Model file for the job. Use its own axes, mm. Face numbers are marked on the shaded views. A direction names the side the tool comes from. Round coordinates to 2 decimals unless told otherwise and drop trailing zeros. Loops run counter-clockwise (first coordinate to the right, second up) from the corner with the lowest first, then second, coordinate; pieces in that order, holes last. Notation, with made-up numbers: (-27, 43) - (31, 43) arc R16 cw to (31, 58) - close; hole circle Ø5 at (77, 21.25). An arc over 180 degrees is marked (long way). Answer as a JSON object with one key per item and string values.
from build123d import *

# Parameters (mm, degrees)
F1_DEPTH = 13
F2_DEPTH = 22
F3_DEPTH = 6
F4_R     = 2
F6_D     = 12
F6_DEPTH = 32
F6_TIP   = 3.6051637142
F7_ANGLE = 180
F9_D     = 12
F9_DEPTH = 35
F9_TIP   = 3.6051637142


with BuildPart() as f1:
    # F0 (on Top) → F1 (new body)
    with BuildSketch(Plane.XY):
        with BuildLine():
            ThreePointArc((26.0064161154, 8), (29.6673325286, 9.0163082132), (32.2804495808, 11.7743529264))
            Line((32.2804495808, 11.7743529264), (84.0861041215, 63.5800074671))
            ThreePointArc((84.0861041215, 63.5800074671), (86.1981822316, 65.1823937822), (87, 67.7093690715))
            Line((87, 67.7093690715), (87, 81))
            ThreePointArc((87, 81), (85.2426406871, 85.2426406871), (81, 87))
            Line((81, 87), (54.36097458, 87))
            ThreePointArc((54.36097458, 87), (58.1513332181, 83.3053678491), (57.5414087508, 78.0475054052))
            Line((57.5414087508, 78.0475054052), (17.2557162005, 37.7618128549))
            ThreePointArc((17.2557162005, 37.7618128549), (11.6428097519, 37.1404544076), (8, 41.455630213))
            Line((8, 41.455630213), (8, 14))
            ThreePointArc((8, 14), (9.7573593129, 9.7573593129), (14, 8))
            Line((14, 8), (26.0064161154, 8))
        make_face()
        with BuildLine():
            ThreePointArc((72.2487373415, 75.7842712475), (75.7842712475, 75.7842712475), (75.7842712475, 72.2487373415))
            Line((75.7842712475, 72.2487373415), (22.7512626585, 19.2157287525))
            ThreePointArc((22.7512626585, 19.2157287525), (19.2157287525, 19.2157287525), (19.2157287525, 22.7512626585))
            Line((19.2157287525, 22.7512626585), (72.2487373415, 75.7842712475))
        make_face(mode=Mode.SUBTRACT)
    extrude(amount=F1_DEPTH)

    # F0 (on Top) → F2 (join)
    with BuildSketch(Plane.XY):
        Polygon((0, 4), (4, 0), (83, 0), (95, 12), (95, 91), (91, 95), (12, 95), (0, 83), align=None)
        with BuildLine():
            Line((84.0861041215, 63.5800074671), (32.2804495808, 11.7743529264))
            ThreePointArc((32.2804495808, 11.7743529264), (29.6673325286, 9.0163082132), (26.0064161154, 8))
            Line((26.0064161154, 8), (14, 8))
            ThreePointArc((14, 8), (9.7573593129, 9.7573593129), (8, 14))
            Line((8, 14), (8, 41.455630213))
            Line((8, 41.455630213), (8, 43.6620265245))
            ThreePointArc((8, 43.6620265245), (6.6419072577, 45.3944081465), (6, 47.5))
            Line((6, 47.5), (6, 72.5))
            ThreePointArc((6, 72.5), (6.5227744249, 74.9494897428), (8, 76.972135955))
            Line((8, 76.972135955), (8, 83.1905249807))
            ThreePointArc((8, 83.1905249807), (9.2565835097, 86.8647595949), (12.5, 89))
            Line((12.5, 89), (37.5, 89))
            ThreePointArc((37.5, 89), (39.9494897428, 88.4772255751), (41.972135955, 87))
            Line((41.972135955, 87), (54.36097458, 87))
            Line((54.36097458, 87), (81, 87))
            ThreePointArc((81, 87), (85.2426406871, 85.2426406871), (87, 81))
            Line((87, 81), (87, 67.7093690715))
            ThreePointArc((87, 67.7093690715), (86.1981822316, 65.1823937822), (84.0861041215, 63.5800074671))
        make_face(mode=Mode.SUBTRACT)
    extrude(amount=F2_DEPTH)

    # F0 (on Top) → F3 (join)
    with BuildSketch(Plane.XY):
        with BuildLine():
            Line((8, 43.6620265245), (8, 41.455630213))
            ThreePointArc((8, 41.455630213), (11.6428097519, 37.1404544076), (17.2557162005, 37.7618128549))
            Line((17.2557162005, 37.7618128549), (57.5414087508, 78.0475054052))
            ThreePointArc((57.5414087508, 78.0475054052), (58.1513332181, 83.3053678491), (54.36097458, 87))
            Line((54.36097458, 87), (41.972135955, 87))
            ThreePointArc((41.972135955, 87), (39.9494897428, 88.4772255751), (37.5, 89))
            Line((37.5, 89), (12.5, 89))
            ThreePointArc((12.5, 89), (9.2565835097, 86.8647595949), (8, 83.1905249807))
            Line((8, 83.1905249807), (8, 76.972135955))
            ThreePointArc((8, 76.972135955), (6.5227744249, 74.9494897428), (6, 72.5))
            Line((6, 72.5), (6, 47.5))
            ThreePointArc((6, 47.5), (6.6419072577, 45.3944081465), (8, 43.6620265245))
        make_face()
    extrude(amount=F3_DEPTH)

    # F4
    f4_edges = [f1.edges().sort_by_distance(p)[0] for p in [
        (51.5, 95, 0),
        (91, 95, 11),
        (95, 91, 11),
        (95, 51.5, 0),
        (93, 93, 0),
        (89, 6, 0),
        (83, 0, 11),
        (95, 12, 11),
        (43.5, 0, 0),
        (4, 0, 11),
        (2, 2, 0),
        (0, 4, 11),
        (0, 43.5, 0),
        (6, 89, 0),
        (0, 83, 11),
        (12, 95, 11),
    ]]
    fillet(f4_edges, radius=F4_R)

    # F6
    with Locations(Plane(origin=(0, 0, 0), x_dir=(0, -1, 0), z_dir=(-1, 0, 0))):
        with Locations((-60, 12)):
            Hole(F6_D / 2, depth=F6_DEPTH)
            with Locations((0, 0, -(F6_DEPTH + F6_TIP / 2))):  # 118° drill point
                Cone(0, F6_D / 2, F6_TIP, mode=Mode.SUBTRACT)


with BuildPart() as f1_1:
    # F7: moved
    add(f1.part.rotate(Axis((43.5, 2, 0), (-1, 0, 0)), F7_ANGLE))

    # F9
    with Locations(Plane.XZ.offset(91)):
        with Locations((25, -12)):
            Hole(F9_D / 2, depth=F9_DEPTH)
            with Locations((0, 0, -(F9_DEPTH + F9_TIP / 2))):  # 118° drill point
                Cone(0, F9_D / 2, F9_TIP, mode=Mode.SUBTRACT)


solid = f1_1.part
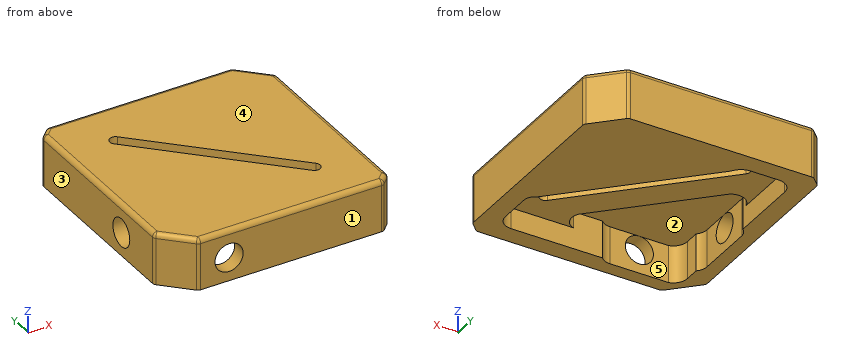
1) Slice it at B-B on x = 46. List the corners of the cut face in (y, z).
Values follow:
{"outline": "(-91, -22) - (-83, -22) - (-83, -6) - (-62.51, -6) - (-62.51, -13) - (-45.54, -13) - (-45.54, 0) - (-89, 0) arc R2 ccw to (-91, -2) - close; (-38.46, -13) - (-21.49, -13) - (-21.49, -22) - (4, -22) - (4, -2) arc R2 ccw to (2, 0) - (-38.46, 0) - close"}
2) Drop a flat-ended pin along its axis: P1, Ø2, axis at x = 23.5, y = -49.5, coming from the -Z side. Give the stop position or say it passes through.
Values follow:
{"P1": "z = -6"}
3) Slice it at C-C on y = -29. List the corners of the cut face in (x, z), then the cut area to 3 significant figures.
Values follow:
{"outline": "(0, -22) - (8, -22) - (8, -13) - (29.46, -13) - (29.46, 0) - (2, 0) arc R2 ccw to (0, -2) - close; (36.54, -13) - (53.51, -13) - (53.51, -22) - (95, -22) - (95, -2) arc R2 ccw to (93, 0) - (36.54, 0) - close", "area": "1,590 mm²"}
4) Probe probe 1 along Y at (x, z) = (48.5, -12); probe 2 along Z at (x, y) = (25, -86.5); probe 3 along Z at (x, y) = (14.5, -61.5). List the from-to ranges inside material, lowest first.
Values follow:
{"probe 1": "-91 to -83, -65.01 to -48.04, -40.96 to 4", "probe 2": "-22 to -18, -6 to 0", "probe 3": "-6 to 0"}
5) Two-plate mould, pull along X, no slides. Class the marked faces 3, 4 and 5: pulls with the +X half, pulls with the -X half, needs draft (parallel to the pull), parting line crosses it, or undercut.
Values follow:
{"face 3": "pulls with the -X half", "face 4": "needs draft", "face 5": "undercut"}
6) Slice it at A-A on z = -4.75. List the corners of the cut face in (x, y), then the cut area to 3 significant figures.
Values follow:
{"outline": "(0, -78.17) arc R2 ccw to (0.59, -79.59) - (11.41, -90.41) arc R2 ccw to (12.83, -91) - (90.17, -91) arc R2 ccw to (91.59, -90.41) - (94.41, -87.59) arc R2 ccw to (95, -86.17) - (95, -8.83) arc R2 ccw to (94.41, -7.41) - (83.59, 3.41) arc R2 ccw to (82.17, 4) - (4.83, 4) arc R2 ccw to (3.41, 3.41) - (0.59, 0.59) arc R2 ccw to (0, -0.83) - close; hole (19.22, -18.75) - (72.25, -71.78) arc R2.5 ccw to (75.78, -68.25) - (22.75, -15.22) arc R2.5 ccw to start", "area": "8,470 mm²"}
7) Slice it at D-D on x = 79. List the corners of the cut face in (y, z).
Values follow:
{"outline": "(-91, -22) - (-83, -22) - (-83, -13) - (-54.49, -13) - (-54.49, -22) - (4, -22) - (4, -2) arc R2 ccw to (2, 0) - (-89, 0) arc R2 ccw to (-91, -2) - close"}
8) Tool access for the marked faces 1 and 2: list every direction of +Z, -Z, +X, -X, +Y, -Y with a clear straight run to the whole face (end or side of a thin tool).
Values follow:
{"face 1": "+Z, -Z, +X, -X, -Y", "face 2": "-Z"}
